```python
from build123d import *

# Parameters (mm, degrees)
SKETCH1_R                = 5
BASE_EXTRUDE_DEPTH       = 100
SKETCH7_OUTSIDE_W        = 32.2
SKETCH7_OUTSIDE_H        = 32.2
SKETCH7_OUTSIDE_R        = 3.5
FRONT_CUT_DEPTH          = 10
FRONT_HOLE_D             = 3
FRONT_HOLE_DEPTH         = 10
FRONT_HOLE_TIP           = 0.901290929
CHAMFER1_SIZE            = 1
KEYWAY_START             = -15
KEYWAY_CUT_DEPTH         = 15
F_4_0_4_BLACK_HOLE_D     = 4
F_4_0_4_BLACK_HOLE_DEPTH = 20
F_4_0_4_BLACK_HOLE_TIP   = 1.201721238


with BuildPart() as part:
    # Sketch1 → Base Extrude (new body)
    with BuildSketch(Plane.XY):
        Circle(SKETCH1_R)
    extrude(amount=BASE_EXTRUDE_DEPTH)

    # Sketch7 outside → Front Cut (cut)
    with BuildSketch(Plane.XY.offset(100)):
        Rectangle(SKETCH7_OUTSIDE_W, SKETCH7_OUTSIDE_H)
        Circle(SKETCH7_OUTSIDE_R, mode=Mode.SUBTRACT)
    extrude(amount=-FRONT_CUT_DEPTH, mode=Mode.SUBTRACT)

    # Front Hole
    with Locations(Plane.XY.offset(100)):
        with Locations((0, 0)):
            Hole(FRONT_HOLE_D / 2, depth=FRONT_HOLE_DEPTH)
            with Locations((0, 0, -(FRONT_HOLE_DEPTH + FRONT_HOLE_TIP / 2))):  # 118° drill point
                Cone(0, FRONT_HOLE_D / 2, FRONT_HOLE_TIP, mode=Mode.SUBTRACT)

    # Chamfer1
    chamfer1_edges = [part.edges().sort_by_distance(p)[0] for p in [
        (-3.5, 0, 100),
    ]]
    chamfer(chamfer1_edges, length=CHAMFER1_SIZE)

    # Keyway → Keyway Cut (cut)
    with BuildSketch(Plane.XY.offset(90).offset(KEYWAY_START)):
        with BuildLine():
            Line((4, 3), (4, -3))
            ThreePointArc((4, -3), (5, 0), (4, 3))
        make_face()
    extrude(amount=KEYWAY_CUT_DEPTH, mode=Mode.SUBTRACT)

    # Ø4.0 (4) Black Hole
    with Locations(Plane(origin=(0, 0, 0), x_dir=(-1, 0, 0), z_dir=(0, 0, -1))):
        with Locations((0, 0)):
            Hole(F_4_0_4_BLACK_HOLE_D / 2, depth=F_4_0_4_BLACK_HOLE_DEPTH)
            with Locations((0, 0, -(F_4_0_4_BLACK_HOLE_DEPTH + F_4_0_4_BLACK_HOLE_TIP / 2))):  # 118° drill point
                Cone(0, F_4_0_4_BLACK_HOLE_D / 2, F_4_0_4_BLACK_HOLE_TIP, mode=Mode.SUBTRACT)


solid = part.part
```
Design review of the part built by this model. Coordinates are the model's own, in mm. A direction names the side the tool comes from. Coordinates: 2 decimals unless noted, no trailing zeros. Loops run counter-clockwise (first coordinate to the right, second up) from the corner with the lowest first, then second, coordinate; pieces in that order, holes last. Notation, with made-up numbers: M -35.75,29.25 L -12.75,29.25 A23 ccw -12.75,48.25 Z; hole C 24.25,77.5 d7. An arc over 180 degrees is marked long. One line per question, with ' | ' between items.
(1) We need section A-A (z = 26.5). Give the boundary of the cut face in (x, y), and give its area (3 significant figures).
Filled in:
outline: C 0,0 d10 | area: 78.5 mm^2
(2) Machinability: for faces 5 (the face through (0, -2, 10)), 6 (the face through (-5, 0, 44)), 7 (the face through (3.233, -1.341, 94.563)), which of the approach directions +Z, -Z, +X, -X, +Y, -Y give a long, thin tool a straight path to every point of the face, cutting with its end or side? Answer none if there is none.
Filled in:
face 5: -Z | face 6: +Z, -Z | face 7: +Z
(3) Wall thickness on probe 1 along Y at (x, z) = (0, 97); probe 2 along X at (y, z) = (0, 14): over which ranges is each line inside the solid? List them lowest first.
Filled in:
probe 1: y = -3.5 to -1.5, 1.5 to 3.5 | probe 2: x = -5 to -2, 2 to 5
(4) For pin 1 Ø3 at (x, y) = (0, 0) entering from -Z; pin 2 Ø1 at (x, z) = (-3.5, 52.5) entering from +Y; pin 3 Ø1.1 at (x, y) = (4.5, -0.5) entering from +Z, all flat-tipped, find the tip position at first contact; note any pin that passes through.
Filled in:
pin 1: stops at z = 20.3 | pin 2: stops at y = 4 | pin 3: stops at z = 90
(5) Draft analysis for pull direction X (two halves, no side actions). For faces 1 (the face through (-4, 0, 90)), 2 (the face through (0.08, -0.34, 20.99)), 3 (the face through (4, 0, 82)), 4 (the face through (1.5, 0.07, 94.93)), state which applies: released by +X, released by -X, zero draft, split by the parting line, or undercut.
Filled in:
face 1: zero draft | face 2: undercut | face 3: released by +X | face 4: undercut
